Check sheet for the drawn part. Datum: minimum x, y, z corner. Units: mm. A direction names the side the tool comes from. Coordinates: 2 decimals unless noted, no trailing zeros. Loops run counter-clockwise (first coordinate to the right, second up) from the corner with the lowest first, then second, coordinate; pieces in that order, holes last. Notation, with made-up numbers: (49, 83.25) -> (61, 83.25) arc R12 cw to (61, 102.25) -> close; hole circle Ø8 at (14.25, 65.25). An arc over 180 degrees is marked (long way). Use CSV: the item, a comma, the result in double quotes. Start each with the question number.
1. Sectioned sample at B-B, the plane y = 5. Record the cut outline in (x, z).
2. Set-up check for the marked faces 1 and 2: record each of +Z, -Z, +X, -X, +Y, -Y from which the full face is reachable in a straight line by a thin tool's end or side.
3. Sectioned sample at C-C, the plane x = 100. Record the cut outline in (y, z), and give its area (3 significant figures).
4. Sectioned sample at D-D, the plane z = 4. Record the cut outline in (x, y), and give its area (3 significant figures).
5. Sectioned sample at A-A, the plane x = 30. Record the cut outline in (y, z).
6. Thickness scan on L1, parallel to Y at x = 30, z = 1.55; L2, parallel to Z at x = 21.5, y = 2; L3, parallel to X at y = 5.75, z = 12.25. Record the ranges inside material, lowest first.
7. Gauge pin test, flat ends, axial feed: pin 1 (1 mm diameter, centred on y = 2.5, z = 7, fed in from +X); pin 2 (2 mm diameter, centred on x = 94, y = 5.5, fed in from +Z). Record the tip position at first contact, or that the pin passes through.
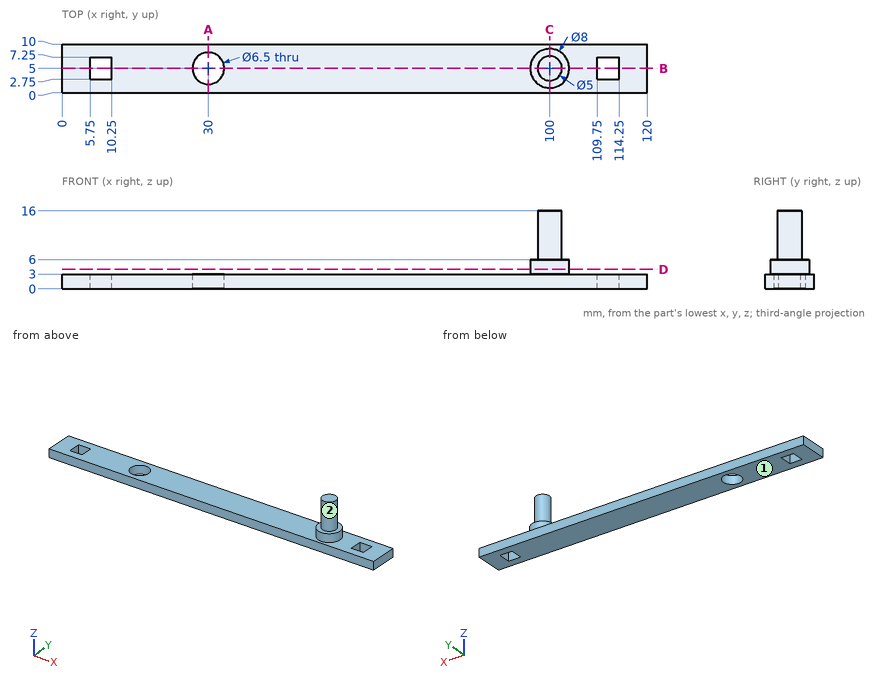
Completed:
1,outline,"(0, 0) -> (5.75, 0) -> (5.75, 3) -> (0, 3) -> close; (10.25, 0) -> (26.75, 0) -> (26.75, 3) -> (10.25, 3) -> close; (33.25, 0) -> (109.75, 0) -> (109.75, 3) -> (104, 3) -> (104, 6) -> (102.5, 6) -> (102.5, 16) -> (97.5, 16) -> (97.5, 6) -> (96, 6) -> (96, 3) -> (33.25, 3) -> close; (114.25, 0) -> (120, 0) -> (120, 3) -> (114.25, 3) -> close"
2,face 1,"-Z, +X, -X, +Y, -Y"
2,face 2,"+Z"
3,outline,"(0, 0) -> (10, 0) -> (10, 3) -> (9, 3) -> (9, 6) -> (7.5, 6) -> (7.5, 16) -> (2.5, 16) -> (2.5, 6) -> (1, 6) -> (1, 3) -> (0, 3) -> close"
3,area,"104 mm²"
4,outline,"circle Ø8 at (100, 5)"
4,area,"50.3 mm²"
5,outline,"(0, 0) -> (1.75, 0) -> (1.75, 3) -> (0, 3) -> close; (8.25, 0) -> (10, 0) -> (10, 3) -> (8.25, 3) -> close"
6,L1,"0 to 1.75, 8.25 to 10"
6,L2,"0 to 3"
6,L3,"97.62 to 102.38"
7,pin 1,"x = 101.5"
7,pin 2,"z = 3"
